```python
from build123d import *

# Parameters (mm, degrees)
SKETCH2_W            = 45
SKETCH2_H            = 45
BOSS_EXTRUDE1_DEPTH  = 4
SKETCH3_R            = 0.75
CUT_EXTRUDE1_DEPTH   = 5
SKETCH4_W            = 12
SKETCH4_H            = 12
CUT_EXTRUDE2_DEPTH   = 5
SKETCH5_W            = 55
SKETCH5_H            = 4
BOSS_EXTRUDE2_DEPTH  = 60.654134022
SKETCH7_W            = 4
SKETCH7_H            = 49
BOSS_EXTRUDE3_DEPTH  = 10
CUT_EXTRUDE6_DEPTH   = 5
BOSS_EXTRUDE4_DEPTH  = 55
SKETCH12_W           = 29.80716229
SKETCH12_H           = 30
CUT_EXTRUDE7_DEPTH   = 50
SCALE2_SCALE         = 2
BOSS_EXTRUDE10_DEPTH = 8
SKETCH29_W           = 121.308268044
SKETCH29_H           = 8
BOSS_EXTRUDE11_DEPTH = 98
SKETCH30_R           = 2.5
CUT_EXTRUDE8_DEPTH   = 98
SKETCH31_R           = 2.5
CUT_EXTRUDE9_DEPTH   = 98
SKETCH32_R           = 4
CUT_EXTRUDE10_DEPTH  = 98
FILLET1_R            = 10


with BuildPart() as part:
    # Sketch2 → Boss-Extrude1 (new body)
    with BuildSketch(Plane(origin=(0, 0, 0), x_dir=(0, 0, -1), z_dir=(1, 0, 0))):
        Rectangle(SKETCH2_W, SKETCH2_H)
    extrude(amount=BOSS_EXTRUDE1_DEPTH)

    # Sketch3 → Cut-Extrude1 (cut)
    with BuildSketch(Plane(origin=(4, 0, 0), x_dir=(0, 0, -1), z_dir=(1, 0, 0))):
        with Locations((-7.762444982, 14.365)):
            Circle(SKETCH3_R)
        with Locations((-7.762444982, -1.135)):
            Circle(SKETCH3_R)
        with Locations((7.737555018, -1.135)):
            Circle(SKETCH3_R)
        with Locations((7.737555018, 14.365)):
            Circle(SKETCH3_R)
    extrude(amount=-CUT_EXTRUDE1_DEPTH, mode=Mode.SUBTRACT)

    # Sketch4 → Cut-Extrude2 (cut)
    with BuildSketch(Plane(origin=(4, 0, 0), x_dir=(0, 0, -1), z_dir=(1, 0, 0))):
        with Locations((0.001587774, 6.615)):
            Rectangle(SKETCH4_W, SKETCH4_H)
    extrude(amount=-CUT_EXTRUDE2_DEPTH, mode=Mode.SUBTRACT)

    # Sketch5 → Boss-Extrude2 (add)
    with BuildSketch(Plane(origin=(0, 0, 0), x_dir=(0, 0, -1), z_dir=(1, 0, 0))):
        with Locations((5, -24.5)):
            Rectangle(SKETCH5_W, SKETCH5_H)
    extrude(amount=BOSS_EXTRUDE2_DEPTH)

    # Sketch7 → Boss-Extrude3 (add)
    with BuildSketch(Plane(origin=(0, 0, -22.5), x_dir=(-1, 0, 0), z_dir=(0, 0, -1))):
        with Locations((-2, -2)):
            Rectangle(SKETCH7_W, SKETCH7_H)
    extrude(amount=BOSS_EXTRUDE3_DEPTH)

    # Sketch9 → Cut-Extrude6 (cut, through all)
    with BuildSketch(Plane(origin=(4, 0, 0), x_dir=(0, 0, -1), z_dir=(1, 0, 0))):
        Polygon((-22.5, 15.5), (-22.5, 22.5), (-15.5, 22.5), align=None)
    extrude(amount=-CUT_EXTRUDE6_DEPTH, mode=Mode.SUBTRACT)

    # Sketch11 → Boss-Extrude4 (add)
    with BuildSketch(Plane.XY.offset(22.5)):
        Polygon((4, -19.5), (7, -22.5), (4, -22.5), align=None)
    extrude(amount=-BOSS_EXTRUDE4_DEPTH)

    # Sketch12 → Cut-Extrude7 (cut, through all)
    with BuildSketch(Plane.XZ.offset(26.5)):
        with Locations((18.903581145, -5)):
            Rectangle(SKETCH12_W, SKETCH12_H)
    extrude(amount=-CUT_EXTRUDE7_DEPTH, mode=Mode.SUBTRACT)


with BuildPart() as part_1:
    # Scale2: scaled about (18.662210537, -12.9832523, -5.287627144)
    add(part.part.scale(SCALE2_SCALE).moved(Location((-18.662210537, 12.9832523, 5.287627144))))

    # Sketch21 → Boss-Extrude10 (add)
    with BuildSketch(Plane(origin=(0, -40.0167477, 0), x_dir=(-1, 0, 0), z_dir=(0, -1, 0))):
        Polygon((10.662210537, -25.287627144), (4.662210537, -25.287627144), (-48.952114042, 11.991594358), (-48.952114042, 34.712372856), (-32.483264947, 34.712372856), (10.662210537, 4.712372856), align=None)
    extrude(amount=-BOSS_EXTRUDE10_DEPTH)

    # Sketch29 → Boss-Extrude11 (add)
    with BuildSketch(Plane.XZ.offset(40.0167477)):
        with Locations((41.991923485, -55.712372856)):
            Rectangle(SKETCH29_W, SKETCH29_H)
    extrude(amount=-BOSS_EXTRUDE11_DEPTH)

    # Sketch30 → Cut-Extrude8 (cut)
    with BuildSketch(Plane(origin=(0, -32.0167477, 0), x_dir=(1, 0, 0), z_dir=(0, 1, 0))):
        with Locations((80.823761479, -27.259651972)):
            Circle(SKETCH30_R)
    extrude(amount=-CUT_EXTRUDE8_DEPTH, mode=Mode.SUBTRACT)

    # Sketch31 → Cut-Extrude9 (cut)
    with BuildSketch(Plane(origin=(0, -32.0167477, 0), x_dir=(1, 0, 0), z_dir=(0, 1, 0))):
        with Locations((80.823761479, 35.016859129)):
            Circle(SKETCH31_R)
    extrude(amount=-CUT_EXTRUDE9_DEPTH, mode=Mode.SUBTRACT)

    # Sketch32 → Cut-Extrude10 (cut)
    with BuildSketch(Plane(origin=(0, 0, -59.712372856), x_dir=(-1, 0, 0), z_dir=(0, 0, -1))):
        with Locations((-89.60887453, 38.7332523)):
            Circle(SKETCH32_R)
        with Locations((-4.609196036, 38.499466475)):
            Circle(SKETCH32_R)
    extrude(amount=-CUT_EXTRUDE10_DEPTH, mode=Mode.SUBTRACT)

    # Fillet1
    fillet1_edges = [part_1.edges().sort_by_distance(p)[0] for p in [
        (102.646057507, 57.9832523, -55.712372856),
    ]]
    fillet(fillet1_edges, radius=FILLET1_R)


solid = part_1.part
```
Input: part model. Units: mm. Frame: model coordinates. A direction names the side the tool comes from. Give positions to 0.01 mm unless a question says otherwise; leave off trailing zeros. Write each loop counter-clockwise with the first axis right and the second up, starting at its lowest first coordinate (ties: lowest second). Pieces come first, ordered by that corner, then holes. Notation, with made-up numbers: (61, 40.25) - (89, 40.25) arc R24 ccw to (89, 52.25) - close; hole circle Ø1 at (53, 35). An arc over 180 degrees is marked (long way). Write item = value, one per line. Start each with the question number.
1. Section query C-C, the plane y = -15.5. Output: boundary loops of the cut face in (x, z), then the cut area to 3 significant figures.
2. First-contact query: pin 1 Ø2 at (y, z) = (40, -29.5) entering from +X; pin 2 Ø9 at (x, y) = (4.61, 38.5) entering from +Z; pin 3 Ø3 at (x, z) = (84.5, 37) entering from +Y. Flat tips, straight axial feed; report the tip coordinate or a pass-through.
3. Ray query, L1, parallel to Z at x = 95, y = 20; L2, parallel to X at y = 14.5, z = 39; L3, parallel to Y at x = 15, z = -41. Return the intervals inside material, ascending.
4. Section query A-A, the plane x = 30.5. Output: boundary loops of the cut face in (y, z).
5. Section query D-D, the plane y = -30. Output: boundary loops of the cut face in (x, z), then the cut area to 3 significant figures.
6. Mould query, pull axis Y, two halves, no side actions, for faces 4 (the cylindrical face through (93.605, 38.909, -55.768)), 5 (the flat face through (-18.662, 10, -4)), 6 (the flat face through (-7.704, -28.975, 37.963)). Classes: released by +Y, released by -Y, zero draft, split by the parting line, or undercut.
7. Access query for faces 1 (the flat face through (-8, -30, 25.288)), 2 (the flat face through (11, -36, -34.712)), 3 (the flat face through (-15, 26, 17.284)). Directions: +Z, -Z, +X, -X, +Y, -Y. A direction counts if a zero-diameter tool reaches every point of the face in a straight line with its end or side. Return the directions, or none.
8. Section query B-B, the plane z = -17. Output: boundary loops of the cut face in (x, y).
Check sheet entries:
q1.outline = (-18.66, -59.71) - (102.65, -59.71) - (102.65, -51.71) - (-10.66, -51.71) - (-10.66, 50.29) - (-18.66, 50.29) - close
q1.area = 1,790 mm2
q2.pin_1 = -10.66
q2.pin_2 = -51.71
q2.pin_3 = -32.02
q3.L1 = -59.71 to -51.71
q3.L2 = -18.66 to -10.66
q3.L3 = -40.02 to -32.02
q4.outline = (-40.02, -59.71) - (57.98, -59.71) - (57.98, -51.71) - (-32.02, -51.71) - (-32.02, -34.71) - (-40.02, -34.71) - close; (-40.02, -33.33) - (-32.02, -33.33) - (-32.02, 0.84) - (-40.02, 0.84) - close; (-40.02, 25.29) - (-32.02, 25.29) - (-32.02, 50.29) - (-40.02, 50.29) - close
q5.outline = (-18.66, -59.71) - (102.65, -59.71) - (102.65, -51.71) - (-6.68, -51.71) - (-6.68, -34.71) - (-10.66, -34.71) - (-10.66, 25.29) - (-6.68, 25.29) - (-6.68, 50.29) - (-18.66, 50.29) - close
q5.area = 1,950 mm2
q6.face_4 = undercut
q6.face_5 = zero draft
q6.face_6 = released by +Y
q7.face_1 = +X, +Y
q7.face_2 = +Y, -Y
q7.face_3 = +X, -X
q8.outline = (-18.66, -40.02) - (-10.66, -40.02) - (-10.66, 57.98) - (-18.66, 57.98) - close; (7.01, -40.02) - (102.65, -40.02) - (102.65, -32.02) - (7.01, -32.02) - close
